Design review of the part built by this model. Coordinates are the model's own, in mm. A direction names the side the tool comes from. Give positions to 0.01 mm unless a question says otherwise; leave off trailing zeros. Order: outer loops, then holes, each group sorted by start corner. A loop starts at its lowest first (then second) coordinate and runs counter-clockwise, first axis right, second up. Notation, with made-up numbers: (52.25, 88) - (107.25, 88) arc R19 cw to (107.25, 98) - close; hole circle Ø4 at (59, 38). An arc over 180 degrees is marked (long way). Write each question's results on one line, items separated by ' | '. Start each with the question number.
```python
from build123d import *

# Parameters (mm, degrees)
F1_DEPTH = 5
F2_R     = 1


with BuildPart() as f1:
    # F0 (on Top) → F1 (new body)
    with BuildSketch(Plane.XY):
        with BuildLine():
            ThreePointArc((4, -0.5), (4.146447, -0.146447), (4.5, 0))
            Line((4.5, 0), (7.496493, 0))
            ThreePointArc((7.496493, 0), (7.850046, -0.146447), (7.996493, -0.5))
            Line((7.996493, -0.5), (7.996493, -2.5))
            ThreePointArc((7.996493, -2.5), (7.930228, -2.747809), (7.74912, -2.92947))
            ThreePointArc((7.74912, -2.92947), (7.566733, -3.112414), (7.5, -3.361974))
            ThreePointArc((7.5, -3.361974), (7.75044, -3.79524), (8.25088, -3.794477))
            ThreePointArc((8.25088, -3.794477), (8.796761, -3.246929), (8.996493, -2.5))
            Line((8.996493, -2.5), (8.996493, -0.5))
            ThreePointArc((8.996493, -0.5), (9.14294, -0.146447), (9.496493, 0))
            Line((9.496493, 0), (15, 0))
            Line((15, 0), (15, 1))
            Line((15, 1), (0, 1))
            Line((0, 1), (0, 0))
            Line((0, 0), (2.5, 0))
            ThreePointArc((2.5, 0), (2.853553, -0.146447), (3, -0.5))
            Line((3, -0.5), (3, -2.5))
            ThreePointArc((3, -2.5), (7.306682, -6.995846), (11.98339, -2.88628))
            ThreePointArc((11.98339, -2.88628), (11.853651, -2.505321), (11.485236, -2.34336))
            ThreePointArc((11.485236, -2.34336), (11.147197, -2.474944), (10.987081, -2.80044))
            ThreePointArc((10.987081, -2.80044), (7.349641, -5.996769), (4, -2.5))
            Line((4, -2.5), (4, -0.5))
        make_face()
    extrude(amount=F1_DEPTH)

    # F2
    f2_edges = [f1.edges().sort_by_distance(p)[0] for p in [
        (15, 0.5, 5),
        (15, 0.5, 0),
        (0, 0.5, 5),
        (0, 0.5, 0),
    ]]
    fillet(f2_edges, radius=F2_R)


solid = f1.part
```
Q1. Insertion check: pin 1 Ø2.5 at (x, z) = (13.5, 2.5) entering from -Y; pin 2 Ø2.5 at (x, z) = (6.5, 3.5) entering from -Y; pin 3 Ø2 at (y, z) = (-1.5, 2) entering from -X; pin 4 Ø1 at (y, z) = (-6, 2) entering from +X. Each pin has a flat end and moves straight along its axis. Give the tip position at first contact, or say it passes through.
Q2. Add section A-A (y = -1.75). Give the boundary of the cut face in (x, z).
Q3. Add section D-D (x = 13.5). Give the boundary of the cut face in (y, z), plus the area to 3 significant figures.
Q4. Draft analysis for pull direction X (two halves, no side actions). For faces 1 (the flat face through (6, 0, 2)), 2 (the flat face through (8.4, -2.4, 0)), 3 (the cylindrical face through (0.285, 0.493, 0.301)), state which applies: pulls with the +X half, pulls with the -X half, needs draft (parallel to the pull), parting line crosses it, or undercut.
Q5. Add section C-C (z = 1.8). Give the boundary of the cut face in (x, y).
Q6. Machinability: for faces 4 (the flat face through (12, 0, 2)), 5 (the flat face through (7.996, -1, 2)), 6 (the flat face through (1, 0, 2)), which of the approach directions +Z, -Z, +X, -X, +Y, -Y give a long, thin tool a straight path to every point of the face, cutting with its end or side? Answer none if there is none.
Q7. Add section B-B (x = 10). Give the boundary of the cut face in (y, z), plus the area to 3 significant figures.
Q8. For line 1 (X direction, y = -3, z = 3.9); line 2 (X direction, y = -2.75, z = 2.5); line 3 (Y direction, x = 12.75, z = 4.65), list the stretches that pass through material, from the lowest coordinate up. Write a range as [from, to].
Verdict:
1) pin 1: stops at y = 0 | pin 2: stops at y = -7 | pin 3: stops at x = 3 | pin 4: stops at x = 10.85
2) outline: (3, 0) - (4, 0) - (4, 5) - (3, 5) - close; (8, 0) - (9, 0) - (9, 5) - (8, 5) - close
3) outline: (0, 0) - (1, 0) - (1, 5) - (0, 5) - close | area: 5.00 mm2
4) face 1: undercut | face 2: needs draft | face 3: pulls with the -X half
5) outline: (0, 0) - (2.5, 0) arc R0.5 cw to (3, -0.5) - (3, -2.5) arc R4.5 ccw to (11.98, -2.89) arc R0.5 ccw to (11.49, -2.34) arc R0.5 ccw to (10.99, -2.8) arc R3.5 cw to (4, -2.5) - (4, -0.5) arc R0.5 cw to (4.5, 0) - (7.5, 0) arc R0.5 cw to (8, -0.5) - (8, -2.5) arc R0.5 cw to (7.75, -2.93) arc R0.5 ccw to (7.5, -3.36) arc R0.5 ccw to (8.25, -3.79) arc R1.5 ccw to (9, -2.5) - (9, -0.5) arc R0.5 cw to (9.5, 0) - (15, 0) - (15, 1) - (0, 1) - close
6) face 4: +Z, -Z, +X | face 5: +Z, -Z | face 6: +Z, -Z, -X, -Y
7) outline: (-6.24, 0) - (-4.95, 0) - (-4.95, 5) - (-6.24, 5) - close; (0, 0) - (1, 0) - (1, 5) - (0, 5) - close | area: 11.5 mm2
8) line 1: x = [3.03, 4.04], [7.66, 8.91], [10.96, 11.97] | line 2: x = [3.01, 4.01], [7.93, 8.98], [10.99, 11.98] | line 3: y = [0, 1]
